For this review, use the dimensioned drawing (mm, ordinates from the lowest corner) and the shaded views. Give positions to 0.01 mm unless a question says otherwise; leave off trailing zeros. Write each loop counter-clockwise with the first axis right and the second up, starting at its lowest first coordinate (ties: lowest second). Pieces come first, ordered by that corner, then holes. Notation, with made-up numbers: (54, 63) -> (95, 63) arc R22 ccw to (95, 93) -> close; hole circle Ø11 at (-27.5, 24). An arc over 180 degrees is marked (long way). Answer as CSV lines item,"result".
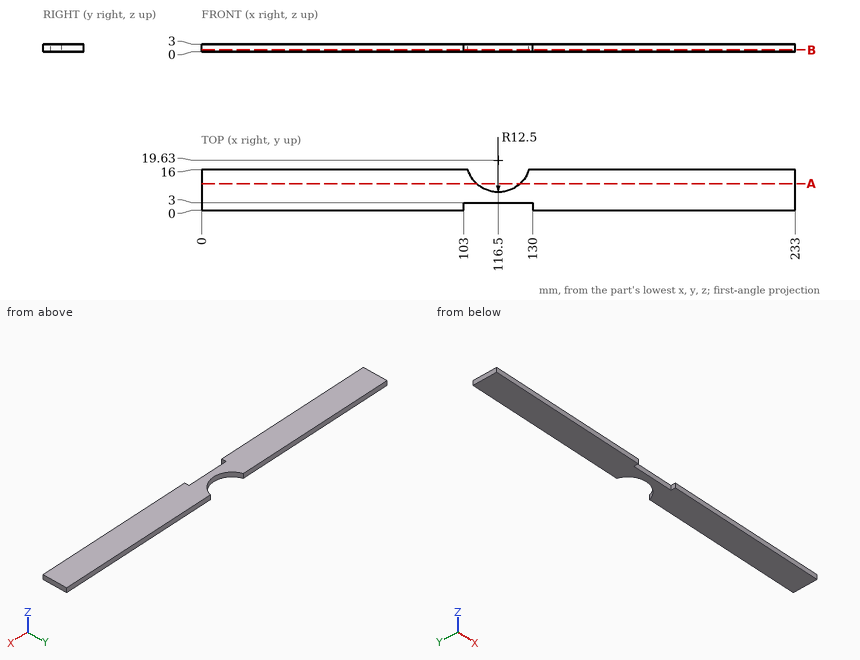
Q1. Add section A-A (y = 10.5). Write out the cut boundary in (x, z), plus the area to 3 significant figures.
Answer block:
outline,"(0, 0) -> (107.96, 0) -> (107.96, 3) -> (0, 3) -> close; (125.04, 0) -> (233, 0) -> (233, 3) -> (125.04, 3) -> close"
area,"648 mm2"
Q2. To check wall thickness, follow probe 1 along X at (y, z) = (1.5, 1.35); probe 2 along X at (y, z) = (12, 0.45); probe 3 along Y at (x, z) = (113.5, 2.2). State the ranges of each line that lie inside material, in increasing order. Write a range as [from, to].
Answer block:
probe 1,"x = [0, 103], [130, 233]"
probe 2,"x = [0, 106.6], [126.4, 233]"
probe 3,"y = [3, 7.5]"
Q3. Add section B-B (z = 0.7). Write out the cut boundary in (x, y).
Answer block:
outline,"(0, 0) -> (103, 0) -> (103, 3) -> (130, 3) -> (130, 0) -> (233, 0) -> (233, 16) -> (128.46, 16) arc R12.5 cw to (104.54, 16) -> (0, 16) -> close"
